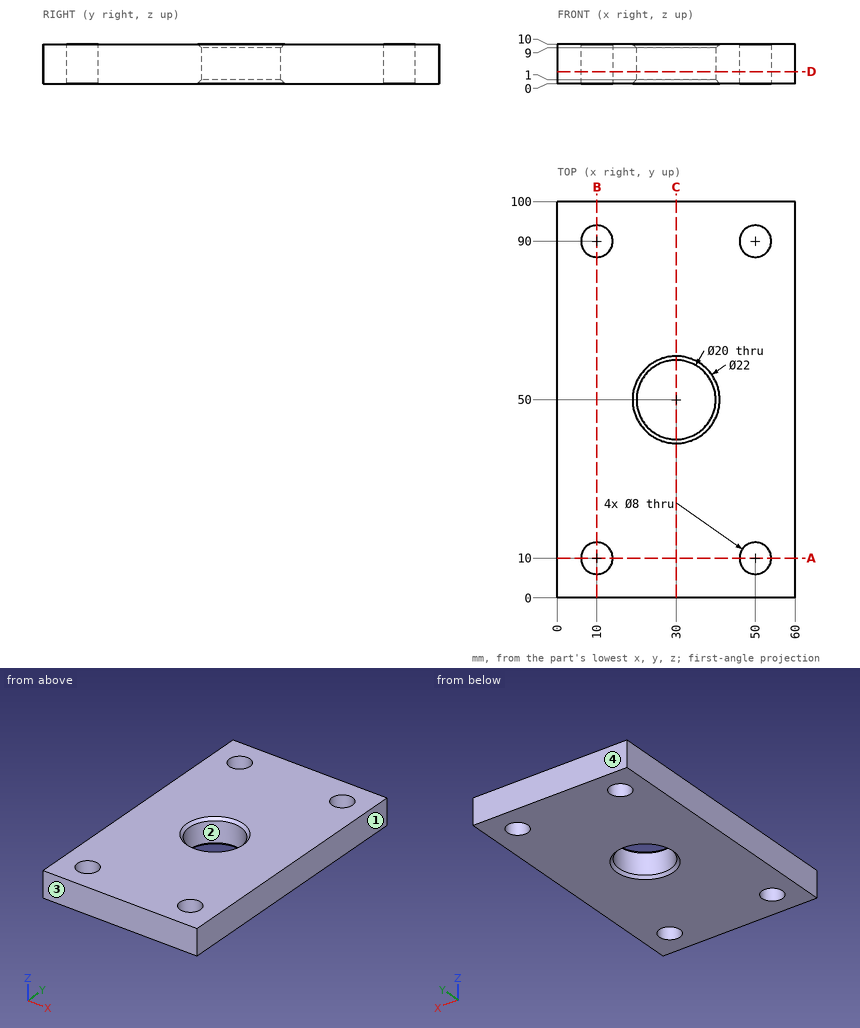
Answer from the drawing. Dimensions are ordinates in mm from the lowest x, y and z of the part. Round coordinates to 2 decimals unless told otherwise and drop trailing zeros. Order: outer loops, then holes, each group sorted by start corner. A loop starts at its lowest first (then second) coordinate and runs counter-clockwise, first axis right, second up.
1) The part is cut by section B-B on x = 10. Write down the section's boundary in (y, z), plus the area to 3 significant figures.
2) The part is cut by section D-D on z = 3. Write down the section's boundary in (x, y), plus the area to 3 significant figures.
3) The mould has two halves that part along Y. Classify the marked faces 1, 2, 3 and 4: released by +Y, released by -Y, zero draft, split by the parting line, or undercut.
4) Straight lines are drawn through the part: L1, parallel to Y at x = 50, z = 4.5; L2, parallel to Y at x = 30, z = 5.75; L3, parallel to X at y = 49.5, z = 4.75. For each, find the intervals that lie inside material, in ascending order.
5) The part is cut by section A-A on y = 10. Write down the section's boundary in (x, z).
6) The part is cut by section C-C on x = 30. Write down the section's boundary in (y, z), plus the area to 3 significant figures.
Resolved:
1. outline: (0, 0) - (6, 0) - (6, 10) - (0, 10) - close; (14, 0) - (86, 0) - (86, 10) - (14, 10) - close; (94, 0) - (100, 0) - (100, 10) - (94, 10) - close
1. area: 840 mm2
2. outline: (0, 0) - (60, 0) - (60, 100) - (0, 100) - close; hole circle Ø8 at (10, 10); hole circle Ø8 at (10, 90); hole circle Ø20 at (30, 50); hole circle Ø8 at (50, 10); hole circle Ø8 at (50, 90)
2. area: 5,480 mm2
3. face 1: zero draft
3. face 2: undercut
3. face 3: released by -Y
3. face 4: released by +Y
4. L1: y = 0 to 6, 14 to 86, 94 to 100
4. L2: y = 0 to 40, 60 to 100
4. L3: x = 0 to 20.01, 39.99 to 60
5. outline: (0, 0) - (6, 0) - (6, 10) - (0, 10) - close; (14, 0) - (46, 0) - (46, 10) - (14, 10) - close; (54, 0) - (60, 0) - (60, 10) - (54, 10) - close
6. outline: (0, 0) - (39, 0) - (40, 1) - (40, 9) - (39, 10) - (0, 10) - close; (60, 1) - (61, 0) - (100, 0) - (100, 10) - (61, 10) - (60, 9) - close
6. area: 798 mm2
